Can you work these out from the model? Positions are in its coordinate system, mm. A direction names the side the tool comes from. Coordinates: 2 decimals unless noted, no trailing zeros. Order: outer loops, then holes, each group sorted by start corner. A loop starts at its lowest first (then second) coordinate and runs counter-clockwise, first axis right, second up. Notation, with made-up numbers: (-11, 85.5) -> (46, 85.5) arc R6 cw to (46, 93.5) -> close; hole circle Ø7 at (22.5, 79). An arc over 180 degrees is marked (long way). Answer as a JSON object with one key per item and string values. Group by question number.
(1) I want a section at C-C, the plane y = -5.5. List the corners of the cut face in (x, z) for me, plus the area to 3 significant figures.
(2) I want a section at D-D, the plane z = -2.25. List the corners of the cut face in (x, y) for me (3 decimals).
(3) I need wall thicknesses on line 1 (Z direction, x = -0.5, y = 2.5); line 2 (Z direction, x = 2, y = -2); line 3 (X direction, y = -6, z = -1.75). Which ranges of each line are inside material? Lowest first, please.
(4) I want a section at A-A, the plane x = 0. List the corners of the cut face in (y, z) for me (3 decimals).
(5) I want a section at B-B, the plane y = -7.25. List the corners of the cut face in (x, z) for me, plus the area to 3 significant figures.
(6) For pin 1 (5 mm diameter, centred on x = 3.5, y = -2.5, fed in from -Z); pin 2 (1.5 mm diameter, centred on y = -4, z = -8, fed in from -X); pin 3 (2.5 mm diameter, centred on y = -4, z = -1.5, fed in from +X); pin 4 (3 mm diameter, centred on x = 1.5, y = 2.5, fed in from +Z), each with a flat end and sliding along its axis, tell me the tip position at first contact or that it passes through.
(7) Which directions (+Z, -Z, +X, -X, +Y, -Y) give clear straight access to the entire face, cutting with the end or side of a thin tool? Please do faces 1 (the cylindrical face through (-0.341, -11.237, 1.041)), 2 (the flat face through (-3.248, -5, -2)), 3 (the flat face through (3.248, -5, -2)).
Autodesk Inventor part; units mm, degrees
ref_plane "YZ Plane" through (0, 0, 0) normal (1, 0, 0) x (0, 1, 0)
ref_plane "XZ Plane" through (0, 0, 0) normal (0, 1, 0) x (-1, 0, 0)
ref_plane "XY Plane" through (0, 0, 0) normal (0, 0, 1) x (1, 0, 0)
sketch "Sketch2" plane through (0, 0, 0) normal (0, 0, 1) x (1, 0, 0)
  arc A0 (3.248, -2.1196) -> (-3.248, -2.1196) centre (0, 0.995) ccw
  line L0 (-3.248, -7.8914) -> (-3.248, -2.1196)
  circle A1 centre (0, -8.005) radius 3.25
  circle A2 centre (0, 0.995) radius 3.25
  line L1 (0, -15.3117) -> (0, 6.7515) construction
  line L2 (3.248, -7.8914) -> (3.248, -2.1196)
  point P0 (0, 0)
  point P1 (-2.9785, -8.0287)
  dimension "d6" = 6.5
  dimension "d7" = 9
  dimension "d8" = 9
extrude "Extrusion1" add sketch "Sketch2" against normal blind 5 contours L2 A1 L0 A0 | A1 | A2
extrude "Extrusion2" add sketch "Sketch2" along normal blind 5 contours A1
sketch "Sketch3" plane through (0, 0, -5) normal (0, 0, -1) x (-1, 0, 0)
  circle A0 centre (0, 0.995) radius 3.25
  point P0 (0, 0)
extrude "Extrusion3" add sketch "Sketch3" along normal blind 5
equation "\"d6\" = R"
equation "\"d7\" = R1"
equation "\"d0\" = thickness"
equation "\"d2\" = thickness"
equation "\"d4\" = thickness"
equation "\"R\" = 6.5"
equation "\"thickness\" = 5"
equation "\"width\" = 6.5"
equation "\"R1\" = 9"
Computed values:
{
 "1": {"outline": "(-3.25, -5) -> (3.25, -5) -> (3.25, 0) -> (2.07, 0) -> (2.07, 5) -> (-2.07, 5) -> (-2.07, 0) -> (-3.25, 0) -> close", "area": "53.2 mm2"},
 "2": {"outline": "(-3.248, -7.891) arc R3.25 ccw (long way) to (3.248, -7.891) -> (3.248, -2.12) arc R4.5 ccw (long way) to (-3.248, -2.12) -> close"},
 "3": {"line 1": "z = -10 to 0", "line 2": "z = -5 to 0", "line 3": "x = -3.25 to 3.25"},
 "4": {"outline": "(-11.255, -5) -> (-2.255, -5) -> (-2.255, -10) -> (4.245, -10) -> (4.245, -5) -> (5.495, -5) -> (5.495, 0) -> (-4.755, 0) -> (-4.755, 5) -> (-11.255, 5) -> close"},
 "5": {"outline": "(-3.25, -5) -> (3.25, -5) -> (3.25, 0) -> (3.16, 0) -> (3.16, 5) -> (-3.16, 5) -> (-3.16, 0) -> (-3.25, 0) -> close", "area": "64.1 mm2"},
 "6": {"pin 1": "stops at z = -10", "pin 2": "passes through", "pin 3": "stops at x = 3.25", "pin 4": "stops at z = 0"},
 "7": {"face 1": "+Z", "face 2": "+Z, -Z, -X, -Y", "face 3": "+Z, -Z, +X, -Y"}
}
